Geometry check sheet. Reference: the model listing, model coordinates, mm. A direction names the side the tool comes from. Round coordinates to 2 decimals unless told otherwise and drop trailing zeros. Write each loop counter-clockwise with the first axis right and the second up, starting at its lowest first coordinate (ties: lowest second). Pieces come first, ordered by that corner, then holes. Notation, with made-up numbers: (17.5, 17.5) -> (44.5, 17.5) arc R12 ccw to (44.5, 30.5) -> close; hole circle Ø3 at (85, -28.75). An arc over 180 degrees is marked (long way). Use a Markdown table: item, result.
```python
from build123d import *

# Parameters (mm, degrees)
SKETCH1_W           = 150
SKETCH1_H           = 100
SKETCH1_R           = 10
BOSS_EXTRUDE1_DEPTH = 20
SKETCH6_R           = 75
BOSS_EXTRUDE2_DEPTH = 20


with BuildPart() as part:
    # Sketch1 → Boss-Extrude1 (new body)
    with BuildSketch(Plane(origin=(0, 0, 0), x_dir=(1, 0, 0), z_dir=(0, 1, 0))):
        with Locations((-11.72985782, -7.612559242)):
            Rectangle(SKETCH1_W, SKETCH1_H)
        with Locations(Location((43.27014218, -37.612559242, 0), (0, 0, 270))):
            Circle(SKETCH1_R, mode=Mode.SUBTRACT)
        with Locations(Location((43.27014218, 22.387440758, 0), (0, 0, 270))):
            Circle(SKETCH1_R, mode=Mode.SUBTRACT)
        with Locations(Location((-66.72985782, 22.387440758, 0), (0, 0, 270))):
            Circle(SKETCH1_R, mode=Mode.SUBTRACT)
        with Locations(Location((-66.72985782, -37.612559242, 0), (0, 0, 270))):
            Circle(SKETCH1_R, mode=Mode.SUBTRACT)
    extrude(amount=BOSS_EXTRUDE1_DEPTH)

    # Sweep1: sweep along a path in Sketch4
    with BuildLine(Plane.ZY.offset(11.72985782)) as sweep1_path:
        Line((-42.387440758, 20), (-42.387440758, 75.147186258))
        ThreePointArc((-42.387440758, 75.147186258), (-37.820212709, 98.1081922), (-24.813847629, 117.573593129))
        Line((-24.813847629, 117.573593129), (40.038966113, 182.426406871))
        ThreePointArc((40.038966113, 182.426406871), (53.045331192, 201.8918078), (57.612559242, 224.852813742))
        Line((57.612559242, 224.852813742), (57.612559242, 280))
    # Sketch5 → Sweep1 (sweep)
    with BuildSketch(Plane(origin=(0, 20, 0), x_dir=(1, 0, 0), z_dir=(0, 1, 0))):
        Polygon((-31.72985782, 42.387440758), (8.27014218, 42.387440758), (8.27014218, 32.387440758), (-6.72985782, 32.387440758), (-6.72985782, 12.387440758), (-16.72985782, 12.387440758), (-16.72985782, 32.387440758), (-31.72985782, 32.387440758), align=None)
    sweep(path=sweep1_path.line)

    # Sketch6 → Boss-Extrude2 (add)
    with BuildSketch(Plane(origin=(0, 280, 0), x_dir=(1, 0, 0), z_dir=(0, 1, 0))):
        with Locations(Location((-11.72985782, -67.612559242, 0), (0, 0, 270))):
            Circle(SKETCH6_R)
        with BuildLine():
            ThreePointArc((-11.72985782, -11.612559242), (-51.327837566, -28.014579495), (-67.72985782, -67.612559242))
            ThreePointArc((-67.72985782, -67.612559242), (-61.72985782, -73.612559242), (-55.72985782, -67.612559242))
            ThreePointArc((-55.72985782, -67.612559242), (-42.842556192, -36.499860869), (-11.72985782, -23.612559242))
            ThreePointArc((-11.72985782, -23.612559242), (-5.72985782, -17.612559242), (-11.72985782, -11.612559242))
        make_face(mode=Mode.SUBTRACT)
        with BuildLine():
            ThreePointArc((-11.72985782, -123.612559242), (27.868121927, -107.210538988), (44.27014218, -67.612559242))
            ThreePointArc((44.27014218, -67.612559242), (38.27014218, -61.612559242), (32.27014218, -67.612559242))
            ThreePointArc((32.27014218, -67.612559242), (19.382840552, -98.725257614), (-11.72985782, -111.612559242))
            ThreePointArc((-11.72985782, -111.612559242), (-17.72985782, -117.612559242), (-11.72985782, -123.612559242))
        make_face(mode=Mode.SUBTRACT)
    extrude(amount=BOSS_EXTRUDE2_DEPTH)


solid = part.part
```
(1) Thickness scan on line 1 (Y direction, x = -67, z = 56.5); line 2 (Y direction, x = -24, z = 34.5); line 3 (Z direction, x = -16, y = 41). Record the ranges inside material, lowest first.
A:
| item | result |
|---|---|
| line 1 | y = 0 to 20, 280 to 300 |
| line 2 | y = 0 to 20, 162.75 to 176.89, 280 to 300 |
| line 3 | z = -42.39 to -12.39 |
(2) Section check C-C on z = 93. Record the cut outline in (x, y).
A:
| item | result |
|---|---|
| outline | (-82.3, 280) -> (24.21, 280) -> (24.21, 300) -> (-82.3, 300) -> close; (38.18, 280) -> (58.84, 280) -> (58.84, 300) -> (38.18, 300) -> close |
(3) Section check A-A on z = 8. Record the cut outline in (x, y), plus the area to 3 significant figures.
A:
| item | result |
|---|---|
| outline | (-86.73, 0) -> (63.27, 0) -> (63.27, 20) -> (-86.73, 20) -> close; (-57.24, 280) -> (33.78, 280) -> (33.78, 300) -> (-57.24, 300) -> close; (-31.73, 136.25) -> (-16.73, 136.25) -> (-16.73, 107.96) -> (-6.73, 107.96) -> (-6.73, 136.25) -> (8.27, 136.25) -> (8.27, 150.39) -> (-31.73, 150.39) -> close |
| area | 5,670 mm2 |
(4) Access from +Z, -Z, +X, -X, +Y, -Y to the whole of each face (thin tool, end or side, straight path). Record for faces 4 (the face through (-11.8, 129.24, 29.28)), 5 (the face through (27.43, 289.86, 107.644)), 6 (the face through (-12, 253, 87.613)), 7 (the face through (-24, 48, -32.387)), 8 (the face through (-24, 253, 67.613)).
A:
| item | result |
|---|---|
| face 4 | +Z, +X, -X |
| face 5 | +Y, -Y |
| face 6 | +Z, +X, -X, -Y |
| face 7 | +Z, -X |
| face 8 | +Z, -X, -Y |
(5) Section check B-B on x = 21.5. Record the cut outline in (y, z), plus the area to 3 significant figures.
A:
| item | result |
|---|---|
| outline | (0, -42.39) -> (20, -42.39) -> (20, 57.61) -> (0, 57.61) -> close; (280, 0.38) -> (300, 0.38) -> (300, 96.45) -> (280, 96.45) -> close; (280, 112.69) -> (300, 112.69) -> (300, 134.85) -> (280, 134.85) -> close |
| area | 4,360 mm2 |
(6) Section check D-D on x = 47.5. Record the cut outline in (y, z), plus the area to 3 significant figures.
A:
| item | result |
|---|---|
| outline | (0, -42.39) -> (20, -42.39) -> (20, -31.45) -> (0, -31.45) -> close; (0, -13.33) -> (20, -13.33) -> (20, 28.55) -> (0, 28.55) -> close; (0, 46.67) -> (20, 46.67) -> (20, 57.61) -> (0, 57.61) -> close; (280, 21.6) -> (300, 21.6) -> (300, 113.62) -> (280, 113.62) -> close |
| area | 3,120 mm2 |
(7) Release check for a two-part mould opening along Z. For faces 1 (the face through (-13, 10, 57.613)), 2 (the face through (-5.73, 289.86, 17.74)), 3 (the face through (-12.01, 201.59, 52.92)) record: +Z half, -Z half, draft (parallel to the pull), parting line (faces both ways), or undercut.
A:
| item | result |
|---|---|
| face 1 | +Z half |
| face 2 | undercut |
| face 3 | -Z half |
(8) Gauge pin test, flat ends, axial feed: pin 1 Ø3 at (x, y) = (-12.5, 60.5) entering from +Z; pin 2 Ø22 at (x, y) = (22, 14) entering from +Z; pin 3 Ø7.5 at (x, y) = (-1.5, 248) entering from +Z; pin 4 Ø2 at (x, z) = (-44.5, 23) entering from +Y. Record the tip position at first contact, or that the pin passes through.
A:
| item | result |
|---|---|
| pin 1 | stops at z = -12.39 |
| pin 2 | stops at z = 57.61 |
| pin 3 | stops at z = 67.61 |
| pin 4 | stops at y = 300 |
